Can you work these out from the drawing? Everything is in mm from the part's minimum corner. A direction names the side the tool comes from. Round coordinates to 2 decimals unless told otherwise and drop trailing zeros. Order: outer loops, then holes, each group sorted by start corner. A loop starts at its lowest first (then second) coordinate and runs counter-clockwise, first axis right, second up. Notation, with made-up numbers: (60.25, 82.25) -> (69.25, 82.25) arc R27 ccw to (69.25, 110.25) -> close; hole circle Ø7 at (69.5, 62.5). An arc over 180 degrees is marked (long way). One line per item, written item: value.
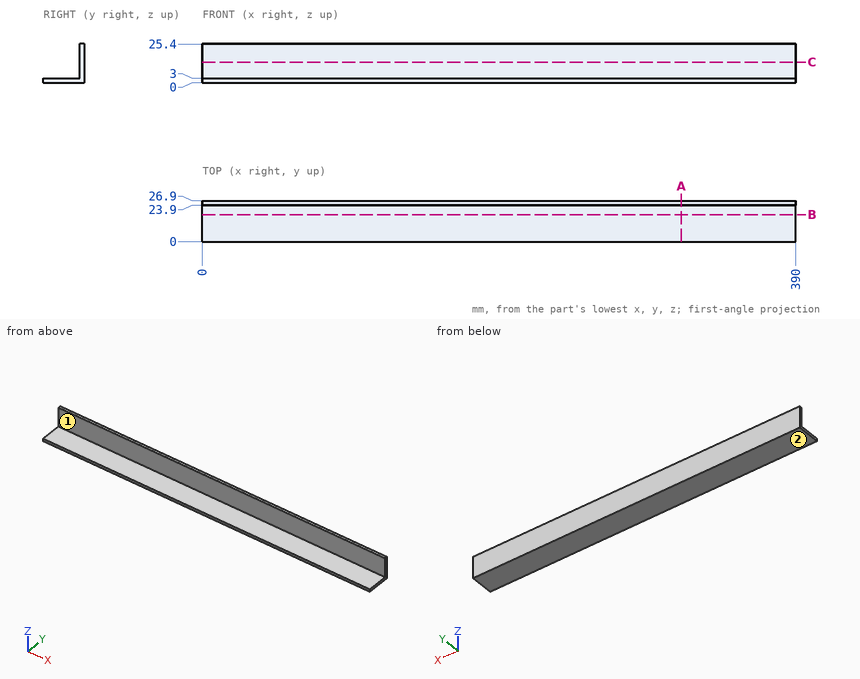
Q1. I want a section at B-B on y = 17.75. List the corners of the cut face in (x, z) for me.
Answers below:
outline: (0, 0) -> (390, 0) -> (390, 3) -> (0, 3) -> close
Q2. Will these pins go through, and if not, where does the flat tip stop? pin 1 Ø5 at (x, y) = (286.5, 3) entering from +Z; pin 2 Ø4 at (x, z) = (47.5, 23) entering from -Y.
Answers below:
pin 1: z = 3
pin 2: y = 23.9
Q3. Please list where these lines run through material, in increasing order: line 1 along Z through (x, y) = (147.5, 8.25); line 2 along Y through (x, z) = (159, 21.5).
Answers below:
line 1: 0 to 3
line 2: 23.9 to 26.9
Q4. On a 3-axis mill with a long thin cutter (end or side, diameter ignored), from which of +Z, -Z, +X, -X, +Y, -Y can I reach the whole of each face in a straight line? I mean the marked faces 1 and 2. Say none if no direction works.
Answers below:
face 1: +Z, +X, -X, -Y
face 2: -Z, +X, -X, +Y, -Y
Q5. I want a section at C-C on z = 13.5. List the corners of the cut face in (x, y) for me.
Answers below:
outline: (0, 23.9) -> (390, 23.9) -> (390, 26.9) -> (0, 26.9) -> close
Q6. I want a section at A-A on x = 315. List the corners of the cut face in (y, z) for me, plus the area to 3 significant figures.
Answers below:
outline: (0, 0) -> (26.9, 0) -> (26.9, 25.4) -> (23.9, 25.4) -> (23.9, 3) -> (0, 3) -> close
area: 148 mm^2
